```python
from build123d import *

# Parameters (mm, degrees)
IZIM1_R                     = 17.5
Y_KSEKLIK_EKSTR_ZYON1_DEPTH = 10
KES_EKSTR_ZYON1_DEPTH       = 3
M4_DI_LI_DELIK1_D           = 3.3
M4_DI_LI_DELIK1_DEPTH       = 8
M4_DI_LI_DELIK1_CSINK_D     = 4.05
M4_DI_LI_DELIK1_CSINK_ANGLE = 90
M4_DI_LI_DELIK1_TIP         = 0.991420021
M4_DI_LI_DELIK2_D           = 3.3
M4_DI_LI_DELIK2_CSINK_D     = 4.05
M4_DI_LI_DELIK2_CSINK_ANGLE = 90
IZIM10_R                    = 1.5
KES_EKSTR_ZYON3_DEPTH       = 26.719642299


with BuildPart() as part:
    # Çizim1 → Yükseklik-Ekstrüzyon1 (new body)
    with BuildSketch(Plane(origin=(0, 0, 0), x_dir=(1, 0, 0), z_dir=(0, 1, 0))):
        with Locations(Location((0, 0, 0), (0, 0, 270))):
            Circle(IZIM1_R)
    extrude(amount=Y_KSEKLIK_EKSTR_ZYON1_DEPTH)

    # Çizim2 → Kes-Ekstrüzyon1 (cut)
    with BuildSketch(Plane(origin=(0, 10, 0), x_dir=(1, 0, 0), z_dir=(0, 1, 0))):
        with BuildLine():
            ThreePointArc((-7.424621202, 7.424621202), (-10.5, 0), (-7.424621202, -7.424621202))
            ThreePointArc((-7.424621202, -7.424621202), (-3.889087297, -7.424621202), (-3.889087297, -3.889087297))
            ThreePointArc((-3.889087297, -3.889087297), (-5.5, 0), (-3.889087297, 3.889087297))
            ThreePointArc((-3.889087297, 3.889087297), (-3.889087297, 7.424621202), (-7.424621202, 7.424621202))
        make_face()
        with BuildLine():
            ThreePointArc((7.424621202, 7.424621202), (10.5, 0), (7.424621202, -7.424621202))
            ThreePointArc((7.424621202, -7.424621202), (3.889087297, -7.424621202), (3.889087297, -3.889087297))
            ThreePointArc((3.889087297, -3.889087297), (5.5, 0), (3.889087297, 3.889087297))
            ThreePointArc((3.889087297, 3.889087297), (3.889087297, 7.424621202), (7.424621202, 7.424621202))
        make_face()
    extrude(amount=-KES_EKSTR_ZYON1_DEPTH, mode=Mode.SUBTRACT)

    # M4 Dişli Delik1
    with Locations(Plane(origin=(0, 0, 0), x_dir=(-1, 0, 0), z_dir=(0, -1, 0))):
        with Locations((0, -12.5), (0, 12.5)):
            CounterSinkHole(M4_DI_LI_DELIK1_D / 2, M4_DI_LI_DELIK1_CSINK_D / 2, depth=M4_DI_LI_DELIK1_DEPTH, counter_sink_angle=M4_DI_LI_DELIK1_CSINK_ANGLE)
            with Locations((0, 0, -(M4_DI_LI_DELIK1_DEPTH + M4_DI_LI_DELIK1_TIP / 2))):  # 118° drill point
                Cone(0, M4_DI_LI_DELIK1_D / 2, M4_DI_LI_DELIK1_TIP, mode=Mode.SUBTRACT)

    # M4 Dişli Delik2 (through all)
    with Locations(Plane(origin=(0, 10, 0), x_dir=(1, 0, 0), z_dir=(0, 1, 0))):
        with Locations((0, 0)):
            CounterSinkHole(M4_DI_LI_DELIK2_D / 2, M4_DI_LI_DELIK2_CSINK_D / 2, counter_sink_angle=M4_DI_LI_DELIK2_CSINK_ANGLE)

    # Çizim10 → Kes-Ekstrüzyon3 (cut, through all)
    with BuildSketch(Plane(origin=(0, 7, 0), x_dir=(1, 0, 0), z_dir=(0, 1, 0))):
        with Locations(Location((-8, 0, 0), (0, 0, 270))):
            Circle(IZIM10_R)
        with Locations(Location((8, 0, 0), (0, 0, 270))):
            Circle(IZIM10_R)
    extrude(amount=-KES_EKSTR_ZYON3_DEPTH, mode=Mode.SUBTRACT)


solid = part.part
```
The listing builds one solid part. Answer for the finished solid, in the listing's coordinates (mm). A direction names the side the tool comes from. Give positions to 0.01 mm unless a question says otherwise; leave off trailing zeros. Loops run counter-clockwise (first coordinate to the right, second up) from the corner with the lowest first, then second, coordinate; pieces in that order, holes last. Notation, with made-up numbers: (25, 73.5) - (83, 73.5) arc R12 ccw to (83, 96.5) - close; hole circle Ø3 at (-13.5, 63). An arc over 180 degrees is marked (long way). Answer as CSV lines item,"result". Start each with the question number.
Item 1: Each of these flat-tipped pins is pushed along its axis until it touches: pin 1 (3.5 mm diameter, centred on x = -8, z = 0, fed in from +Y); pin 2 (1.5 mm diameter, centred on y = 6.5, z = 4, fed in from -X); pin 3 (1.5 mm diameter, centred on x = -3, y = 6, fed in from -Z). Where does it stop, or does it pass through?
Item 2: A cutting plane is placed at C-C on x = -8. Determine the outline of the cut face in (y, z).
Item 3: The mould has two halves that part along X. Classify faces 1 (the face through (-10.5, 8.5, -0.1)), 2 (the face through (-4, 10, 0)): +X half, -X half, draft (parallel to the pull), parting line (faces both ways), or undercut.
Item 4: A cutting plane is placed at B-B on z = 0. Determine the outline of the cut face in (x, y) (3 decimals).
Item 5: For faces 3 (the face through (6.536, 3.549, -0.325)), 4 (the face through (-0.4, 4.2, 14.1)), 5 (the face through (-5.5, 8.5, 0.1)), determine the directions among +Z, -Z, +X, -X, +Y, -Y from which every point of the face is accessible in a straight line to the end or side of a thin tool.
Item 6: A cutting plane is placed at A-A on y = 1.5. Determine the outline of the cut face in (x, z).
Item 7: Find the intervals of material crossed by line 1 (X direction, y = 4.75, z = 0.5); line 2 (X direction, y = 8, z = -1.5); line 3 (Y direction, x = 5, z = -6), in increasing order. Write a range as from..to.
Item 8: A cutting plane is placed at D-D on z = 6. Determine the outline of the cut face in (x, y).
Found:
1,pin 1,"stops at y = 7"
1,pin 2,"stops at x = -17.2"
1,pin 3,"stops at z = -17.35"
2,outline,"(0, -15.56) - (10, -15.56) - (10, -6.8) - (7, -6.8) - (7, -1.5) - (0, -1.5) - close; (0, 1.5) - (7, 1.5) - (7, 6.8) - (10, 6.8) - (10, 15.56) - (0, 15.56) - close"
3,face 1,"undercut"
3,face 2,"draft"
4,outline,"(-17.5, 0) - (-9.5, 0) - (-9.5, 7) - (-10.5, 7) - (-10.5, 10) - (-17.5, 10) - close; (-6.5, 0) - (-1.65, 0) - (-1.65, 9.625) - (-2.025, 10) - (-5.5, 10) - (-5.5, 7) - (-6.5, 7) - close; (1.65, 0) - (6.5, 0) - (6.5, 7) - (5.5, 7) - (5.5, 10) - (2.025, 10) - (1.65, 9.625) - close; (9.5, 0) - (17.5, 0) - (17.5, 10) - (10.5, 10) - (10.5, 7) - (9.5, 7) - close"
5,face 3,"+Y, -Y"
5,face 4,"-Y"
5,face 5,"+Y"
6,outline,"circle Ø35 at (0, 0); hole circle Ø3 at (-8, 0); hole circle Ø3.3 at (0, -12.5); hole circle Ø3.3 at (0, 0); hole circle Ø3.3 at (0, 12.5); hole circle Ø3 at (8, 0)"
7,line 1,"x = -17.49..-9.41, -6.59..-1.57, 1.57..6.59, 9.41..17.49"
7,line 2,"x = -17.44..-10.39, -5.29..-0.69, 0.69..5.29, 10.39..17.44"
7,line 3,"y = 0..7"
8,outline,"(-16.44, 0) - (16.44, 0) - (16.44, 10) - (8.62, 10) - (8.62, 7) - (3.18, 7) - (3.18, 10) - (-3.18, 10) - (-3.18, 7) - (-8.62, 7) - (-8.62, 10) - (-16.44, 10) - close"
